from build123d import *

# Parameters (mm, degrees)
F2_R     = 2.5
F3_DEPTH = 60


with BuildPart() as f1:
    # F0 (on Front) → F1 (revolve)
    with BuildSketch(Plane.XZ):
        Polygon((50, 0), (0, 60), (0, 0), align=None)
    revolve(axis=Axis((0, 0, 30), (0, 0, -1)))

    # F2 (on Top) → F3 (cut)
    with BuildSketch(Plane.XY):
        Circle(F2_R)
    extrude(amount=F3_DEPTH, mode=Mode.SUBTRACT)

    # F4 (on Front) → F5 (revolve, cut)
    with BuildSketch(Plane.XZ):
        Polygon((0, 55), (0, 0), (45, 0), align=None)
    revolve(axis=Axis((0, 0, 27.5), (0, 0, 1)), mode=Mode.SUBTRACT)


solid = f1.part
For this review, take the finished solid that the model builds, in its own axes (mm). Give positions to 0.01 mm unless a question says otherwise; leave off trailing zeros. Loops run counter-clockwise (first coordinate to the right, second up) from the corner with the lowest first, then second, coordinate; pieces in that order, holes last.
Item 1: Insertion check: pin 1 (12 mm diameter, centred on x = 25, y = 18, fed in from +Z); pin 2 (8 mm diameter, centred on x = 35, y = 1, fed in from +Z); pin 3 (4 mm diameter, centred on x = -7, y = -16, fed in from +Z). Each pin has a flat end and moves straight along its axis. Give the tip position at first contact, or say it passes through.
Item 2: Take a section at D-D, the plane z = 29. State the section outline as (x, y) points.
Item 3: Take a section at A-A, the plane x = 0. State the section outline as (y, z) points.
Item 4: Take a section at C-C, the plane z = 39. State the section outline as (x, y) points.
Item 5: For line 1 along X through (y, z) = (19, 5); line 2 along X through (y, z) = (0, 55.9); line 3 along Y through (x, z) = (0, 54), list the stretches that pass through material, from the lowest coordinate up.
Item 6: Draft analysis for pull direction Y (two halves, no side actions). For faces 1 (the flat face through (41, -19, 0)), 2 (the conical face through (14.65, -4.61, 41.57)), 3 (the cylindrical face through (-0.54, -2.44, 54.44)), state which applies: +Y half, -Y half, draft (parallel to the pull), parting line (faces both ways), or undercut.
Calculated:
1. pin 1: stops at z = 30.23
1. pin 2: stops at z = 22.78
1. pin 3: stops at z = 41.44
2. outline: circle Ø51.67 at (0, 0); hole circle Ø42.55 at (0, 0)
3. outline: (-50, 0) - (-45, 0) - (-2.5, 51.94) - (-2.5, 57) - close; (2.5, 51.94) - (45, 0) - (50, 0) - (2.5, 57) - close
4. outline: circle Ø35 at (0, 0); hole circle Ø26.18 at (0, 0)
5. line 1: x = -41.71 to -36.23, 36.23 to 41.71
5. line 2: x = -3.42 to -2.5, 2.5 to 3.42
5. line 3: y = -5 to -2.5, 2.5 to 5
6. face 1: draft
6. face 2: parting line
6. face 3: undercut
